Input: part model. Units: mm. Frame: model coordinates. A direction names the side the tool comes from. Give positions to 0.01 mm unless a question says otherwise; leave off trailing zeros. Write each loop counter-clockwise with the first axis right and the second up, starting at its lowest first coordinate (ties: lowest second). Pieces come first, ordered by that corner, then holes. Notation, with made-up numbers: (-31, -30.5) - (-25, -30.5) arc R23 cw to (-25, -14.5) - close; hole circle Ø11 at (61, -24). An arc over 180 degrees is marked (long way). Answer as CSV lines item,"result".
```python
from build123d import *

# Parameters (mm, degrees)
SKETCH1_W           = 41.5
SKETCH1_H           = 22.75
BOSS_EXTRUDE1_DEPTH = 1.5
SKETCH1_3_W         = 4.75
SKETCH1_3_H         = 12
SKETCH1_3_W_2       = 4
SKETCH1_3_H_2       = 3
BOSS_EXTRUDE2_DEPTH = 2


with BuildPart() as part:
    # Sketch1 → Boss-Extrude1 (new body)
    with BuildSketch(Plane.XY):
        with Locations((20.75, 11.375)):
            Rectangle(SKETCH1_W, SKETCH1_H)
    extrude(amount=BOSS_EXTRUDE1_DEPTH)

    # Sketch1_3 → Boss-Extrude2 (add)
    with BuildSketch(Plane.XY):
        with Locations((22.125, 9)):
            Rectangle(SKETCH1_3_W, SKETCH1_3_H)
        with Locations((7.5, 13.75)):
            Rectangle(SKETCH1_3_W_2, SKETCH1_3_H_2)
    extrude(amount=-BOSS_EXTRUDE2_DEPTH)


solid = part.part
```
Item 1: Ray query, line 1 (X direction, y = 14, z = -0.3); line 2 (X direction, y = 4, z = -1.05); line 3 (Z direction, x = 15, y = 18.75). Return the intervals inside material, ascending. Write a range as from..to.
The answers:
line 1,"5.5..9.5, 19.75..24.5"
line 2,"19.75..24.5"
line 3,"0..1.5"
Item 2: Cut plane B-B on y = 3.75. Return the cut outline in (x, z), plus the area to 4 significant figures.
The answers:
outline,"(0, 0) - (19.75, 0) - (19.75, -2) - (24.5, -2) - (24.5, 0) - (41.5, 0) - (41.5, 1.5) - (0, 1.5) - close"
area,"71.75 mm²"
Item 3: Reachability of faces 1 (the face through (7, 12.25, -1)), 2 (the face through (19.75, 9, -1)), 3 (the face through (5.5, 14, -1)), 4 (the face through (22, 3, -1)), 5 (the face through (22, 15, -1)) from +Z, -Z, +X, -X, +Y, -Y: full face, straight path, thin tool, end or side. Return the list, or none.
The answers:
face 1,"-Z, -X, -Y"
face 2,"-Z, +Y, -Y"
face 3,"-Z, -X, +Y, -Y"
face 4,"-Z, +X, -X, -Y"
face 5,"-Z, +X, +Y"
Item 4: Cut plane D-D on y = 14. Return the cut outline in (x, z).
The answers:
outline,"(0, 0) - (5.5, 0) - (5.5, -2) - (9.5, -2) - (9.5, 0) - (19.75, 0) - (19.75, -2) - (24.5, -2) - (24.5, 0) - (41.5, 0) - (41.5, 1.5) - (0, 1.5) - close"
Item 5: Contact query for flat-ended pins moving along their axis: pin 1 (2 mm diameter, centred on y = 9.5, z = -1.5, fed in from +X); pin 2 (1.6 mm diameter, centred on y = 14.5, z = -1, fed in from -X); pin 3 (2 mm diameter, centred on x = 10.5, y = 15.5, fed in from -Z). Output: stop coordinate, or through.
The answers:
pin 1,"x = 24.5"
pin 2,"x = 5.5"
pin 3,"z = 0"
Item 6: Cut plane C-C on x = 24. Return the cut outline in (y, z).
The answers:
outline,"(0, 0) - (3, 0) - (3, -2) - (15, -2) - (15, 0) - (22.75, 0) - (22.75, 1.5) - (0, 1.5) - close"
Item 7: Cut plane A-A on z = -0.45. Return the cut outline in (x, y).
The answers:
outline,"(5.5, 12.25) - (9.5, 12.25) - (9.5, 15.25) - (5.5, 15.25) - close; (19.75, 3) - (24.5, 3) - (24.5, 15) - (19.75, 15) - close"
